Source: CAD feature listing. Evaluate the final solid. Frame: model axes, mm. Face numbers are marked on the shaded views. A direction names the side the tool comes from. Coordinates: 2 decimals unless noted, no trailing zeros. Loops run counter-clockwise (first coordinate to the right, second up) from the corner with the lowest first, then second, coordinate; pieces in that order, holes last. Notation, with made-up numbers: (71.5, 10) -> (98.5, 10) arc R24 ccw to (98.5, 22) -> close; hole circle Ø8 at (-13.5, 85.5). An arc over 180 degrees is marked (long way). Answer as CSV lines item,"result".
Autodesk Inventor part; units mm, degrees
ref_plane "YZ Plane" through (0, 0, 0) normal (1, 0, 0) x (0, 1, 0)
ref_plane "XZ Plane" through (0, 0, 0) normal (0, 1, 0) x (-1, 0, 0)
ref_plane "XY Plane" through (0, 0, 0) normal (0, 0, 1) x (1, 0, 0)
sketch "Sketch1" plane through (0, 0, 0) normal (0, 1, 0) x (-1, 0, 0)
  line L0 (-24, 63) -> (24, 63)
  line L1 (24, 63) -> (24, -63)
  line L2 (24, -63) -> (-24, -63)
  line L3 (-24, -63) -> (-24, 63)
  line L4 (-24, 63) -> (24, -63) construction
  line L5 (24, 63) -> (-24, -63) construction
  line L6 (-20, 59) -> (20, 59) construction
  line L7 (20, 59) -> (20, -59) construction
  line L8 (20, -59) -> (-20, -59) construction
  line L9 (-20, -59) -> (-20, 59) construction
  line L10 (-20, 59) -> (20, -59) construction
  line L11 (20, 59) -> (-20, -59) construction
  circle A0 centre (20, 59) radius 1.55
  circle A1 centre (20, -59) radius 1.55
  circle A2 centre (-20, -59) radius 1.55
  circle A3 centre (-20, 59) radius 1.55
  point P0 (0, 0)
  dimension "d0" = 126
  dimension "d1" = 48
  dimension "d2" = 3.1
  dimension "d3" = 4
  dimension "d4" = 4
  dimension "d5" = 3.1
  dimension "d6" = 3.1
  dimension "d7" = 3.1
extrude "Extrusion1" add sketch "Sketch1" along normal blind 1.6
fillet "Fillet1" radius 5 4 edges at (24, 0.8, -63) (-24, 0.8, -63) (24, 0.8, 63) (-24, 0.8, 63)
sketch "Sketch2" plane through (0, 0, 0) normal (0, -1, 0) x (1, 0, 0)
  circle A0 centre (20, 59) radius 1.55
  circle A1 centre (20, 59) radius 2.1
  circle A2 centre (20, 59) radius 3.5
  line L0 (0, 0) -> (23.8307, 0) construction
  line L1 (0, 0) -> (0, 62.8307) construction
  circle A3 centre (20, -59) radius 1.55
  circle A4 centre (20, -59) radius 2.1
  circle A5 centre (20, -59) radius 3.5
  circle A6 centre (-20, 59) radius 1.55
  circle A7 centre (-20, 59) radius 2.1
  circle A8 centre (-20, 59) radius 3.5
  circle A9 centre (-20, -59) radius 1.55
  circle A10 centre (-20, -59) radius 2.1
  circle A11 centre (-20, -59) radius 3.5
  point P0 (-23.8307, 0)
  dimension "d11" = 4.2
  dimension "d12" = 7
extrude "Extrusion2" add sketch "Sketch2" along normal blind 6.5 contours A2 | A5 | A8 | A11
sketch "Sketch3" plane through (20, -6.5, -59) normal (0, -1, 0) x (1, 0, 0)
  line L0 (-47, 125) -> (7, 125)
  line L1 (7, 125) -> (7, -7)
  line L2 (7, -7) -> (-47, -7)
  line L3 (-47, -7) -> (-47, 125)
  line L4 (-47, 125) -> (7, -7) construction
  line L5 (7, 125) -> (-47, -7) construction
  line L6 (4, 117) -> (4, 1)
  line L7 (-39, 122) -> (-1, 122)
  point P0 (-20, 59)
  dimension "d17" = 3
  dimension "d18" = 3
extrude "Extrusion3" add sketch "Sketch3" along normal blind 2
sketch "Sketch4" plane through (20, -6.5, -59) normal (0, 1, 0) x (1, 0, 0)
  line L0 (-47, 7) -> (7, 7)
  line L1 (7, -125) -> (-47, -125)
  line L2 (-47, -125) -> (-47, 7)
  line L3 (-47, 7) -> (7, 7)
  line L4 (7, 7) -> (7, -125)
  line L5 (7, -125) -> (-47, 7) construction
  line L6 (-47, -125) -> (7, 7) construction
  line L7 (5, -123) -> (-45, -123)
  line L8 (-45, -123) -> (-45, 5)
  line L9 (-45, 5) -> (5, 5)
  line L10 (5, 5) -> (5, -123)
  line L11 (5, -123) -> (-45, 5) construction
  line L12 (-45, -123) -> (5, 5) construction
  point P0 (-20, -59)
  dimension "d21" = 2
  dimension "d22" = 2
extrude "Extrusion4" add sketch "Sketch4" along normal blind 24
sketch "Sketch5" plane through (-25, -6.5, 64) normal (1, 0, 0) x (0, 0, -1)
  circle A0 centre (110.2, 15.2) radius 4
  line L0 (6, 6.5) -> (122, 6.5)
  point P0 (64, 6.5)
  point P1 (1, 8.1)
  point P2 (127, 8.1)
  point P3 (108.5902, 6.5)
  point P4 (111.8098, 6.5)
  dimension "d25" = 8.7
  dimension "d27" = 16.8
  dimension "d28" = 8
extrude "Extrusion5" cut sketch "Sketch5" against normal blind 15.5
sketch "Sketch6" plane through (25, -6.5, -64) normal (-1, 0, 0) x (0, 0, 1)
  line L0 (28.9, 21.7) -> (44.6, 21.7)
  line L1 (44.6, 21.7) -> (44.6, 8.1)
  line L2 (44.6, 8.1) -> (28.9, 8.1)
  line L3 (28.9, 8.1) -> (28.9, 21.7)
  line L4 (122, 8.1) -> (6, 8.1)
  point P0 (64, 6.5)
  point P1 (1, 8.1)
  dimension "d31" = 43.6
  dimension "d32" = 15.7
  dimension "d33" = 13.6
extrude "Extrusion6" cut sketch "Sketch6" against normal blind 15.5
fillet "Fillet2" radius 1 4 edges at (26, 1.6, -35.1) (26, 1.6, -19.4) (26, 15.2, -19.4) (26, 15.2, -35.1)
sketch "Sketch7" plane through (-27, -8.5, -66) normal (-1, 0, 0) x (0, 0, 1)
  line L0 (86.3, 29.1) -> (100.3, 29.1)
  line L1 (100.3, 29.1) -> (100.3, 19.1)
  line L2 (100.3, 19.1) -> (86.3, 19.1)
  line L3 (86.3, 19.1) -> (86.3, 29.1)
  line L4 (86.3, 29.1) -> (100.3, 19.1) construction
  line L5 (100.3, 29.1) -> (86.3, 19.1) construction
  line L6 (8, 10.1) -> (124, 10.1)
  point P0 (66, 8.5)
  point P1 (93.3, 24.1)
  point P2 (129, 10.1)
  dimension "d37" = 14
  dimension "d38" = 10
  dimension "d39" = 35.7
  dimension "d40" = 14
extrude "Extrusion7" cut sketch "Sketch7" against normal blind 15.5
sketch "Sketch8" plane through (0, 1.6, 0) normal (0, 1, 0) x (1, 0, 0)
  line L0 (-24, 63) -> (24, 63)
  line L1 (24, 63) -> (24, -63)
  line L2 (24, -63) -> (-24, -63)
  line L3 (-24, -63) -> (-24, 63)
  line L4 (-24, 63) -> (24, -63) construction
  line L5 (24, 63) -> (-24, -63) construction
  line L6 (24, -58) -> (24, 58)
  line L7 (19, 63) -> (-19, 63)
  point P0 (0, 0)
extrude "Extrusion8" cut sketch "Sketch8" against normal blind 1.6
fillet "Fillet3" radius 1.5 4 edges at (-23.5, -6.5, -59) (16.5, -6.5, -59) (16.5, -6.5, 59) (-23.5, -6.5, 59)
fillet "Fillet4" radius 3 4 edges at (25, 5.5, -64) (25, 5.5, 64) (-25, 5.5, 64) (-25, 5.5, -64)
fillet "Fillet5" radius 4 4 edges at (-27, 4.5, 66) (-27, 4.5, -66) (27, 4.5, -66) (27, 4.5, 66)
equation "\"d5\" = d2"
equation "\"d6\" = d2"
equation "\"d7\" = d2"
properties part number "Control_PCB_enclosure"
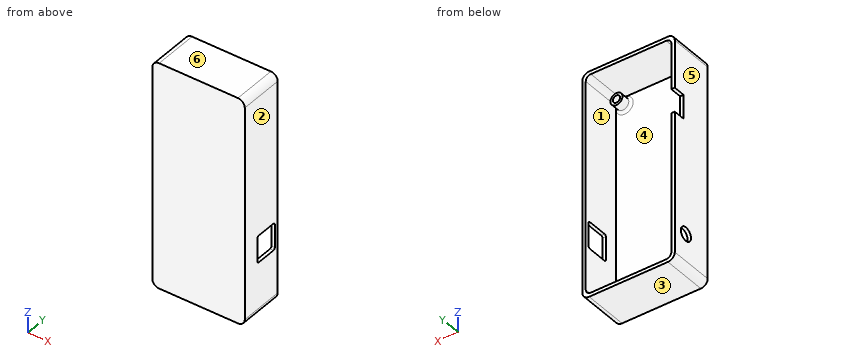
(1) Draft query along Z for the marked faces 3, 4, 5 and 6. Return one class per face: released by +Z, released by -Z, zero draft, split by the parting line, or undercut.
Computed values:
face 3,"released by -Z"
face 4,"undercut"
face 5,"zero draft"
face 6,"released by +Z"
(2) Cut plane B-B (z = -27.5). Return the cut outline in (x, y).
Computed values:
outline,"(-27, -8.5) -> (27, -8.5) -> (27, 1.6) -> (25, 1.6) -> (25, -6.5) -> (-25, -6.5) -> (-25, 17.5) -> (-27, 17.5) -> close; (25, 15.2) -> (27, 15.2) -> (27, 17.5) -> (25, 17.5) -> close"
(3) Pin query (flat end, axial travel): pin 1 Ø5.5 at (x, z) = (20.5, 57.5) entering from +Y; pin 2 Ø3 at (y, z) = (13, -26.5) entering from +X; pin 3 Ø1.6 at (x, y) = (25.5, 9.5) entering from +Z. Return the tip coordinate at first contact, or that it passes through.
Computed values:
pin 1,"y = 0"
pin 2,"x = -25"
pin 3,"z = 65.62"
(4) Access query for the marked faces 1 and 2. Directions: +Z, -Z, +X, -X, +Y, -Y. A direction counts if a zero-diameter tool reaches every point of the face in a straight line with its end or side. Return the directions, or none.
Computed values:
face 1,"+Y"
face 2,"+Z, -Z, +X, +Y, -Y"
(5) Cut plane D-D (z = 9). Return the cut outline in (x, y).
Computed values:
outline,"(-27, -8.5) -> (27, -8.5) -> (27, 17.5) -> (25, 17.5) -> (25, -6.5) -> (-25, -6.5) -> (-25, 17.5) -> (-27, 17.5) -> close"
(6) Cut plane A-A (y = 8.7). Return the cut outline in (x, z).
Computed values:
outline,"(-27, -62) arc R4 ccw to (-23, -66) -> (23, -66) arc R4 ccw to (27, -62) -> (27, -35.1) -> (25, -35.1) -> (25, -61) arc R3 cw to (22, -64) -> (-22, -64) arc R3 cw to (-25, -61) -> (-25, -50.2) -> (-27, -50.2) -> close; (-27, -42.2) -> (-25, -42.2) -> (-25, 61) arc R3 cw to (-22, 64) -> (22, 64) arc R3 cw to (25, 61) -> (25, -19.4) -> (27, -19.4) -> (27, 62) arc R4 ccw to (23, 66) -> (-23, 66) arc R4 ccw to (-27, 62) -> close"
(7) Material intervals for L1, parallel to Z at x = 20, y = -3; L2, parallel to Z at x = 14.5, y = 16.25; L3, parallel to X at y = 4, z = 12, sorted ascending. Write a range as [from, to].
Computed values:
L1,"[-66, -64], [-62.5, -61.1], [-56.9, -55.5], [55.5, 56.9], [61.1, 62.5], [64, 66]"
L2,"[-66, -64], [64, 66]"
L3,"[-27, -25], [25, 27]"
